from build123d import *

# Parameters (mm, degrees)
BOSS_EXTRUDE1_DEPTH = 0.7
FILLET1_R           = 5
FILLET2_R           = 5
FILLET3_R           = 3
SCALE1_SCALE        = 1.2


with BuildPart() as part:
    # Sketch1 → Boss-Extrude1 (new body)
    with BuildSketch(Plane(origin=(0, 0, 0), x_dir=(1, 0, 0), z_dir=(0, 1, 0))):
        with BuildLine():
            ThreePointArc((0, 0), (10.674582486, 2.159113438), (21.303319094, -0.215426558))
            ThreePointArc((21.303319094, -0.215426558), (18.980175942, -13.538262848), (10.41005245, -24))
            ThreePointArc((10.41005245, -24), (1.872716321, -13.445396703), (0, 0))
        make_face()
    extrude(amount=BOSS_EXTRUDE1_DEPTH)

    # Fillet1
    fillet1_edges = [part.edges().sort_by_distance(p)[0] for p in [
        (21.303319094, 0.35, 0.215426558),
    ]]
    fillet(fillet1_edges, radius=FILLET1_R)

    # Fillet2
    fillet2_edges = [part.edges().sort_by_distance(p)[0] for p in [
        (0, 0.35, 0),
    ]]
    fillet(fillet2_edges, radius=FILLET2_R)

    # Fillet3
    fillet3_edges = [part.edges().sort_by_distance(p)[0] for p in [
        (10.41005245, 0.35, 24),
    ]]
    fillet(fillet3_edges, radius=FILLET3_R)


with BuildPart() as part_1:
    # Scale1: scaled about (10.489972613, 0.35, 8.803486941)
    add(part.part.scale(SCALE1_SCALE).moved(Location((-2.097994523, -0.07, -1.760697388))))


solid = part_1.part
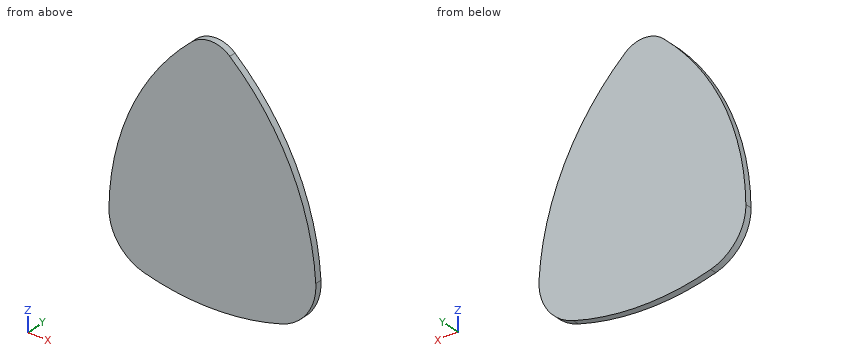
For this review, take the finished solid that the model builds, in its own axes (mm). Round coordinates to 2 decimals unless told otherwise and drop trailing zeros. Loops run counter-clockwise (first coordinate to the right, second up) from the corner with the lowest first, then second, coordinate; pieces in that order, holes last. Notation, with made-up numbers: (67, -20.75) - (108, -20.75) arc R9 cw to (108, -7.75) - close; hole circle Ø3 at (24, 41). An arc over 180 degrees is marked (long way). Answer as CSV lines item,"result".
(1) Insertion check: P1, Ø12, axis at x = 3, z = 21, coming from the -Y side. The pin has a flat end and moves straight along its axis. Give the tip position at first contact, or say it passes through.
Checked values:
P1,"stops at y = -0.07"
(2) Consider section A-A on z = 17.5. Give the boundary of the cut face in (x, y).
Checked values:
outline,"(1.72, -0.07) - (19.1, -0.07) - (19.1, 0.77) - (1.72, 0.77) - close"
(3) Consider section B-B on x = 6. Give the boundary of the cut face in (y, z).
Checked values:
outline,"(-0.07, -4.04) - (0.77, -4.04) - (0.77, 23.22) - (-0.07, 23.22) - close"
(4) Wall thickness on line 1 (X direction, y = 0.65, z = 16); line 2 (Z direction, x = 6, y = 0); line 3 (Z direction, x = 19.5, y = 0.5): over which ranges is each line inside the solid? List them lowest first.
Checked values:
line 1,"x = 0.91 to 19.94"
line 2,"z = -4.04 to 23.22"
line 3,"z = -3 to 16.8"
